from build123d import *

# Parameters (mm, degrees)
BASPROSKE_W                  = 20
BASPROSKE_H                  = 33.75
BASE_REVOLVE_ANGLE           = 134
BASE_REVOLVE_OTHER_WAY_ANGLE = 11
TOOTHCUT_DEPTH               = 52.750603861
TEETHCUTS_COUNT              = 25
TEETHCUTS_ANGLE              = 345.6
BORSKE_R                     = 7.5
BORE_DEPTH                   = 50.000508
BOSS_EXTRUDE1_DEPTH          = 20
SKETCH5_R                    = 7.5
CUT_EXTRUDE1_DEPTH           = 20
FILLET1_R                    = 10
FILLET2_R                    = 10
SCALE1_SCALE                 = 0.8


with BuildPart() as part:
    # BasProSke → Base-Revolve (revolve)
    with BuildSketch(Plane(origin=(0, 0, 0), x_dir=(1, 0, 0), z_dir=(0, 1, 0))):
        with Locations((10, 16.875)):
            Rectangle(BASPROSKE_W, BASPROSKE_H)
    revolve(axis=Axis((-10, 0, 0), (1, 0, 0)), revolution_arc=BASE_REVOLVE_ANGLE)

    # BasProSke → Base-Revolve other way (revolve)
    with BuildSketch(Plane(origin=(0, 0, 0), x_dir=(1, 0, 0), z_dir=(0, 1, 0))):
        with Locations((10, 16.875)):
            Rectangle(BASPROSKE_W, BASPROSKE_H)
    revolve(axis=Axis((-10, 0, 0), (-1, 0, 0)), revolution_arc=BASE_REVOLVE_OTHER_WAY_ANGLE)

    # TooCutSke → ToothCut (cut, through all)
    with BuildSketch(Plane(origin=(0, 0, 0), x_dir=(0, 0, -1), z_dir=(1, 0, 0))):
        with BuildLine():
            ThreePointArc((1.187856988, 28.098903391), (0, 28.124), (-1.187856988, 28.098903391))
            ThreePointArc((-1.187856988, 28.098903391), (-2.083835169, 31.109603364), (-3.702102288, 33.801870579))
            ThreePointArc((-3.702102288, 33.801870579), (0, 34.004), (3.702102288, 33.801870579))
            ThreePointArc((3.702102288, 33.801870579), (2.083835169, 31.109603364), (1.187856988, 28.098903391))
        make_face()
    toothcut = extrude(amount=TOOTHCUT_DEPTH, mode=Mode.SUBTRACT)

    # TeethCuts: ToothCut ×25 about axis
    teethcuts_axis = Axis((-10, 0, 0), (1, 0, 0))
    for i in range(1, TEETHCUTS_COUNT):
        add(toothcut.rotate(teethcuts_axis, i * TEETHCUTS_ANGLE / (TEETHCUTS_COUNT - 1)), mode=Mode.SUBTRACT)

    # BorSke → Bore (cut, symmetric)
    with BuildSketch(Plane(origin=(0, 0, 0), x_dir=(0, 0, -1), z_dir=(1, 0, 0))):
        Circle(BORSKE_R)
    extrude(amount=BORE_DEPTH, both=True, mode=Mode.SUBTRACT)

    # Sketch4 → Boss-Extrude1 (add)
    with BuildSketch(Plane(origin=(20, 0, 0), x_dir=(0, 0, -1), z_dir=(1, 0, 0))):
        with BuildLine():
            Line((-67.553619374, 29.467732547), (-20.230712545, -19.536572011))
            ThreePointArc((-20.230712545, -19.536572011), (7.987647554, -26.965846223), (27.607282907, -5.366312186))
            Line((27.607282907, -5.366312186), (7.362203876, -1.431067465))
            ThreePointArc((7.362203876, -1.431067465), (-3.578690702, -6.591128345), (-5.209937778, 5.395048503))
            Line((-5.209937778, 5.395048503), (-47.322906829, 49.004304558))
            Line((-47.322906829, 49.004304558), (-67.553619374, 29.467732547))
        make_face()
    extrude(amount=-BOSS_EXTRUDE1_DEPTH)

    # Sketch5 → Cut-Extrude1 (cut)
    with BuildSketch(Plane(origin=(20, 0, 0), x_dir=(0, 0, -1), z_dir=(1, 0, 0))):
        with Locations((-48.755033471, 30.244271049)):
            Circle(SKETCH5_R)
    extrude(amount=-CUT_EXTRUDE1_DEPTH, mode=Mode.SUBTRACT)

    # Fillet1
    fillet1_edges = [part.edges().sort_by_distance(p)[0] for p in [
        (10, 49.004304558, 47.322906829),
    ]]
    fillet(fillet1_edges, radius=FILLET1_R)

    # Fillet2
    fillet2_edges = [part.edges().sort_by_distance(p)[0] for p in [
        (10, 29.467732547, 67.553619374),
    ]]
    fillet(fillet2_edges, radius=FILLET2_R)


with BuildPart() as part_1:
    # Scale1: scaled about (10, 7.017353876, 11.436425522)
    add(part.part.scale(SCALE1_SCALE).moved(Location((2, 1.403470775, 2.287285104))))


solid = part_1.part
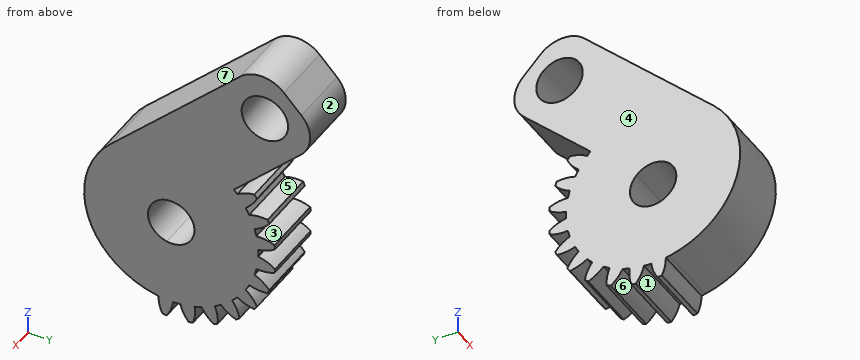
Can you work these out from the model? Positions are in its coordinate system, mm. Face numbers are marked on the shaded views. A direction names the side the tool comes from. Give positions to 0.01 mm unless a question says otherwise; leave off trailing zeros. Loops run counter-clockwise (first coordinate to the right, second up) from the corner with the lowest first, then second, coordinate; pieces in that order, holes last. Notation, with made-up numbers: (-29, 58.25) - (-14, 58.25) arc R4 cw to (-14, 64.25) - close; hole circle Ø2 at (67.5, -28.75). An arc over 180 degrees is marked (long way). One line per item, written item: value.
(1) I need wall thicknesses on line 1 along Z through (x, y) = (14, 18); line 2 along Y through (x, z) = (14.5, 4); line 3 along Y through (x, z) = (4.75, 36). Which ranges of each line are inside material? Lowest first, please.
Verdict:
line 1: -18.81 to -15.12, -12.9 to 17.48, 18.31 to 49.59
line 2: -21.03 to -4.35, 7.15 to 26.39
line 3: 3.93 to 22.77, 28.43 to 36.01
(2) If we section it at D-D, the plane z = 19.5: List the corners of the cut face in (x, y) for me.
Verdict:
outline: (2, -13.16) - (18, -13.16) - (18, 19.23) - (2, 19.23) - close
(3) On a 3-axis mill with a long thin cutter (end or side, diameter ignored), from which of +Z, -Z, +X, -X, +Y, -Y can I reach the whole of each face in a straight line? I mean the marked faces 5, 6 and 7. Say none if no direction works.
Verdict:
face 5: +X, -X
face 6: -Z, +X, -X
face 7: +Z, +X, -X, -Y
(4) If we section it at C-C, the plane x = 17: State how many separate pieces and enclosed holes the cut face has, plus the area to 3 significant figures.
Verdict:
separate pieces: 1
enclosed holes: 2
area: 2,290 mm^2
(5) If we section it at B-B, the plane y = -6.5: List the corners of the cut face in (x, z) for me.
Verdict:
outline: (2, -18.78) - (18, -18.78) - (18, 25.93) - (2, 25.93) - close
(6) If we mould it in two halves opening along Z, with no side actions, what happens to the marked faces 1, 2, 3 and 4? For each: released by +Z, released by -Z, zero draft, split by the parting line, or undercut.
Verdict:
face 1: released by -Z
face 2: split by the parting line
face 3: undercut
face 4: zero draft
(7) If we section it at A-A, the plane z = 37: List the corners of the cut face in (x, y) for me, plus the area to 3 significant figures.
Verdict:
outline: (2, 4.96) - (18, 4.96) - (18, 21.41) - (2, 21.41) - close; (2, 29.79) - (18, 29.79) - (18, 36.56) - (2, 36.56) - close
area: 371 mm^2
(8) I'm going to push flat-ended pins straight in: pin 1 (6 mm diameter, centred on x = 15.5, y = 25, fed in from +Z); pin 2 (1 mm diameter, centred on x = 8.5, y = 27.5, fed in from +Z); pin 3 (4 mm diameter, centred on x = 16, z = 29.5, fed in from -Y); pin 4 (3 mm diameter, centred on x = 5, z = -16.5, fed in from +Y). Where does each tip first touch, or does it pass through?
Verdict:
pin 1: z = 53.02
pin 2: z = 52.7
pin 3: y = -4.88
pin 4: y = 19.02
